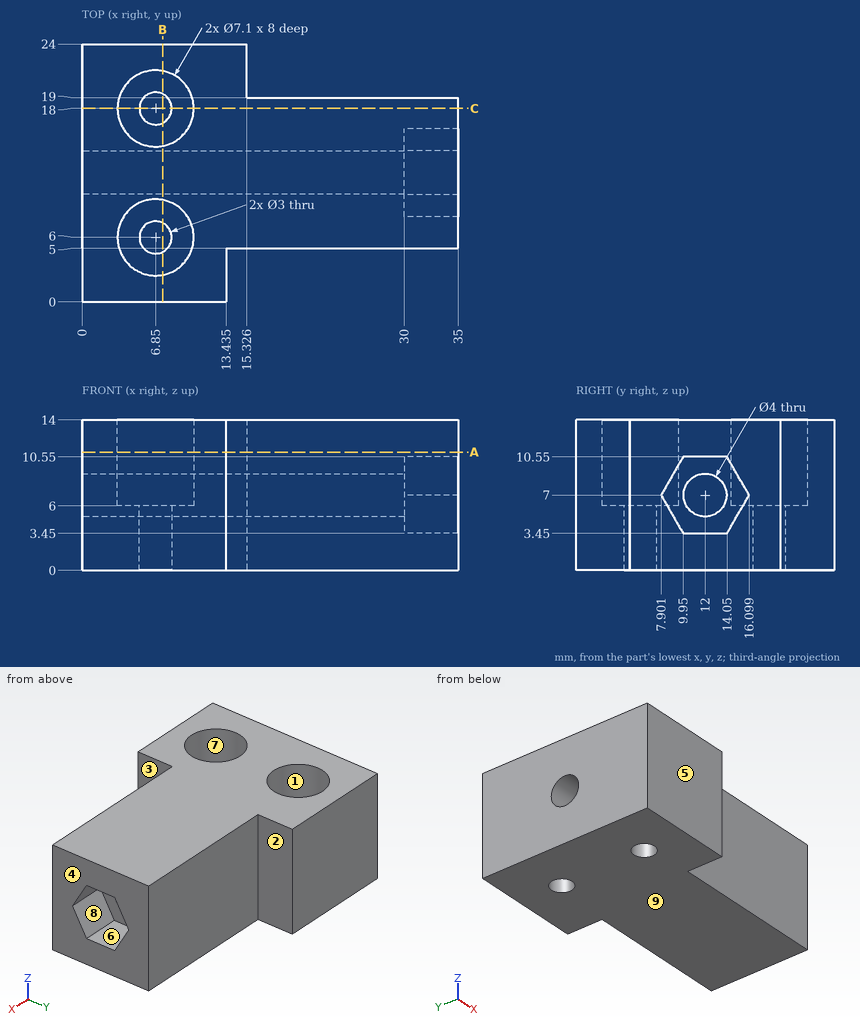
Study the drawing (mm; zero at the part's minimum x, y, z) and answer. A direction names the side the tool comes from. Round coordinates to 2 decimals unless told otherwise and drop trailing zeros. Write each loop counter-clockwise with the first axis right and the second up, starting at its lowest first coordinate (ties: lowest second). Pieces come first, ordered by that corner, then holes. Notation, with made-up numbers: (-19, 3.25) -> (39, 3.25) arc R9 cw to (39, 20.25) -> close; hole circle Ø3 at (66, 32). An arc over 180 degrees is marked (long way). Write item = value, one per line.
1) Straight lines are drawn through the part: line 1 along Y through (x, z) = (5, 8.5) (1 decimal); line 2 along Y through (x, z) = (10.5, 7); line 3 along Z through (x, y) = (7, 8.5). For each, find the intervals that lie inside material, in ascending order. Write a range as [from, to].
Check values:
line_1 = [0, 3], [9, 10.7], [13.3, 15], [21, 24]
line_2 = [0, 10], [14, 24]
line_3 = [0, 6]
2) Which of the six approach directions +Z, -Z, +X, -X, +Y, -Y give full straight-line access (tool end or side, diameter ignored) to the marked faces 1, 2, 3, 4 and 5?
Check values:
face_1 = +Z
face_2 = +Z, -Z, +X, +Y
face_3 = +Z, -Z, +X, -Y
face_4 = +Z, -Z, +X, +Y, -Y
face_5 = +Z, -Z, +X, -X, -Y
3) Section A-A on z = 11 is taken. Give the number of separate pieces and of enclosed holes in the cut face.
Check values:
separate_pieces = 1
enclosed_holes = 2
4) Section C-C on y = 18 is taken. Write down the section's boundary in (x, z), plus the area to 3 significant figures.
Check values:
outline = (0, 0) -> (5.35, 0) -> (5.35, 6) -> (3.3, 6) -> (3.3, 14) -> (0, 14) -> close; (8.35, 0) -> (35, 0) -> (35, 14) -> (10.4, 14) -> (10.4, 6) -> (8.35, 6) -> close
area = 415 mm²
5) Section B-B on x = 7.5 is taken. Write down the section's boundary in (y, z), plus the area to 3 significant figures.
Check values:
outline = (0, 0) -> (4.65, 0) -> (4.65, 6) -> (2.51, 6) -> (2.51, 14) -> (0, 14) -> close; (7.35, 0) -> (16.65, 0) -> (16.65, 6) -> (14.51, 6) -> (14.51, 14) -> (9.49, 14) -> (9.49, 6) -> (7.35, 6) -> close; (19.35, 0) -> (24, 0) -> (24, 14) -> (21.49, 14) -> (21.49, 6) -> (19.35, 6) -> close; hole circle Ø4 at (12, 7)
area = 179 mm²
6) For a pull along Z with two mould halves and no side action, classify the marked faces 6, 7, 8 and 9 as released by +Z, released by -Z, zero draft, split by the parting line, or undercut.
Check values:
face_6 = undercut
face_7 = zero draft
face_8 = undercut
face_9 = released by -Z
7) Given pin 1 (5 mm diameter, centred on x = 6.85, y = 18, fed in from +Z); pin 2 (7 mm diameter, centred on x = 30, z = 8.5, fed in from +Y); pin 3 (4 mm diameter, centred on y = 2, z = 4.5, fed in from +X) (1 decimal), each flat-ended and moving along its own axis, determine where each tip first touches the part or whether it passes through.
Check values:
pin_1 = 6
pin_2 = 19
pin_3 = 13.4
